For this review, take the finished solid that the model builds, in its own axes (mm). A direction names the side the tool comes from. Give positions to 0.01 mm unless a question says otherwise; leave off trailing zeros. Write each loop counter-clockwise with the first axis right and the second up, starting at its lowest first coordinate (ties: lowest second). Pieces come first, ordered by that corner, then holes.
1) We need section B-B on x = 16. Give the boundary of the cut face in (y, z).
2) Machinability: for faces 5 (the face through (40, 5, 49)), 6 (the face through (-50, 5, 0)), which of the approach directions +Z, -Z, +X, -X, +Y, -Y give a long, thin tool a straight path to every point of the face, cutting with its end or side? Answer none if there is none.
3) We need section C-C on z = 14. Give the boundary of the cut face in (x, y), and give its area (3 significant figures).
4) We need section A-A on y = 5. Give the boundary of the cut face in (x, z).
5) For P1, Ø1.5, axis at x = 18, y = 6.5, coming from the +Z side, flat-tipped, find the tip position at first contact; note if it passes through.
6) Wall thickness on line 1 along X through (y, z) = (9.25, 50.5); line 2 along Z through (x, y) = (35, 3.5): over which ranges is each line inside the solid? List them lowest first.
7) Draft analysis for pull direction Y (two halves, no side actions). For faces 1 (the face through (18, 0, 4)), 2 (the face through (-6, 5, 5)), 3 (the face through (-36.73, 3.85, -0.07)), 4 (the face through (18, 10, 4)), state which applies: pulls with the +Y half, pulls with the -Y half, needs draft (parallel to the pull), parting line crosses it, or undercut.
from build123d import *

# Parameters (mm, degrees)
Y_KSEKLIK_EKSTR_ZYON1_DEPTH = 10
IZIM2_R                     = 3
KES_EKSTR_ZYON1_DEPTH       = 113.249721603
IZIM3_R                     = 3
KES_EKSTR_ZYON2_DEPTH       = 139.293166859


with BuildPart() as part:
    # Çizim1 → Yükseklik-Ekstrüzyon1 (new body)
    with BuildSketch(Plane(origin=(0, 0, 0), x_dir=(1, 0, 0), z_dir=(0, 1, 0))):
        Polygon((-50, -5), (40, -5), (40, -95), (50, -95), (50, -10), (50, 5), (18.191830665, 5), (-50, 5), align=None)
    extrude(amount=Y_KSEKLIK_EKSTR_ZYON1_DEPTH)

    # Çizim2 → Kes-Ekstrüzyon1 (cut, through all)
    with BuildSketch(Plane(origin=(0, 0, -5), x_dir=(-1, 0, 0), z_dir=(0, 0, -1))):
        with Locations((33.959177931, 5)):
            Circle(IZIM2_R)
    extrude(amount=-KES_EKSTR_ZYON1_DEPTH, mode=Mode.SUBTRACT)

    # Çizim3 → Kes-Ekstrüzyon2 (cut, through all)
    with BuildSketch(Plane(origin=(50, 0, 0), x_dir=(0, 0, -1), z_dir=(1, 0, 0))):
        with Locations((-69.652523483, 5)):
            Circle(IZIM3_R)
    extrude(amount=-KES_EKSTR_ZYON2_DEPTH, mode=Mode.SUBTRACT)


solid = part.part
Results list:
1. outline: (0, -5) - (10, -5) - (10, 5) - (0, 5) - close
2. face 5: +Z, -X, +Y, -Y
2. face 6: +Z, -Z, -X, +Y, -Y
3. outline: (40, 0) - (50, 0) - (50, 10) - (40, 10) - close
3. area: 100 mm2
4. outline: (-50, -5) - (-36.96, -5) - (-36.96, 5) - (-50, 5) - close; (-30.96, -5) - (50, -5) - (50, 66.65) - (40, 66.65) - (40, 5) - (-30.96, 5) - close; (40, 72.65) - (50, 72.65) - (50, 95) - (40, 95) - close
5. P1: stops at z = 5
6. line 1: x = 40 to 50
6. line 2: z = -5 to 5
7. face 1: pulls with the -Y half
7. face 2: needs draft
7. face 3: undercut
7. face 4: pulls with the +Y half
